Geometry check sheet. Reference: the model listing, model coordinates, mm. Round coordinates to 2 decimals unless told otherwise and drop trailing zeros. Order: outer loops, then holes, each group sorted by start corner. A loop starts at its lowest first (then second) coordinate and runs counter-clockwise, first axis right, second up. Notation, with made-up numbers: (6.25, 85) - (37.25, 85) arc R23 cw to (37.25, 113) - close; hole circle Ø1 at (-4, 59.25). An arc over 180 degrees is marked (long way). One line per question, with ' | ' between items. Start each with the question number.
Q1. Sectioned sample at C-C, the plane z = -30. Enter the section's corners in (x, y), then the cut area to 3 significant figures.
Q2. Sectioned sample at A-A, the plane z = 0. Enter the section's corners in (x, y).
Q3. Sectioned sample at B-B, the plane x = 0. Enter the section's corners in (y, z).
Q4. Material ranges on line 1 along X through (y, z) = (1.8, 0); line 2 along X through (y, z) = (7.55, 0); line 3 along Z through (x, y) = (3.5, 2.5), recorded low to high.
Q5. Sectioned sample at D-D, the plane y = 8.25. Enter the section's corners in (x, z).
Q6. Gauge pin test, flat ends, axial feed: P1, Ø1.5, axis at x = -22.5, y = 1.5, coming from the -Z side; P2, Ø4, axis at x = -14.5, y = 8, coming from the -Z side; P3, Ø1, axis at x = 32.5, y = 3, coming from the -Z side. Record the tip position at first contact, or that the pin passes through.
```python
from build123d import *

# Parameters (mm, degrees)
SKETCH_1_R          = 42.5
EXTRUDE_1_DEPTH     = 10
SKETCH_2_R          = 7
CUT_EXTRUDE_1_DEPTH = 6
SKETCH_3_R          = 2.5
CUT_EXTRUDE_2_DEPTH = 6


with BuildPart() as part:
    # Эскиз1 → Вытянуть1 (new body)
    with BuildSketch(Plane(origin=(0, 0, 0), x_dir=(1, 0, 0), z_dir=(0, 1, 0))):
        with Locations(Location((0, 0, 0), (0, 0, 270))):
            Circle(SKETCH_1_R)
    extrude(amount=EXTRUDE_1_DEPTH)

    # Эскиз2 → Вырез-Вытянуть1 (cut)
    with BuildSketch(Plane.XZ):
        with Locations(Location((-29.48960133, 0, 0), (0, 0, 270))):
            Circle(SKETCH_2_R)
        with Locations(Location((0, 29.48960133, 0), (0, 0, 270))):
            Circle(SKETCH_2_R)
        with Locations(Location((29.48960133, 0, 0), (0, 0, 270))):
            Circle(SKETCH_2_R)
        with Locations(Location((0, -29.48960133, 0), (0, 0, 270))):
            Circle(SKETCH_2_R)
    extrude(amount=-CUT_EXTRUDE_1_DEPTH, mode=Mode.SUBTRACT)

    # Эскиз3 → Вырез-Вытянуть2 (cut)
    with BuildSketch(Plane.XZ.offset(-6)):
        with Locations(Location((-29.48960133, 0, 0), (0, 0, 270))):
            Circle(SKETCH_3_R)
        with Locations(Location((0, 29.48960133, 0), (0, 0, 270))):
            Circle(SKETCH_3_R)
        with Locations(Location((29.48960133, 0, 0), (0, 0, 270))):
            Circle(SKETCH_3_R)
        with Locations(Location((0, -29.48960133, 0), (0, 0, 270))):
            Circle(SKETCH_3_R)
    extrude(amount=-CUT_EXTRUDE_2_DEPTH, mode=Mode.SUBTRACT)


solid = part.part
```
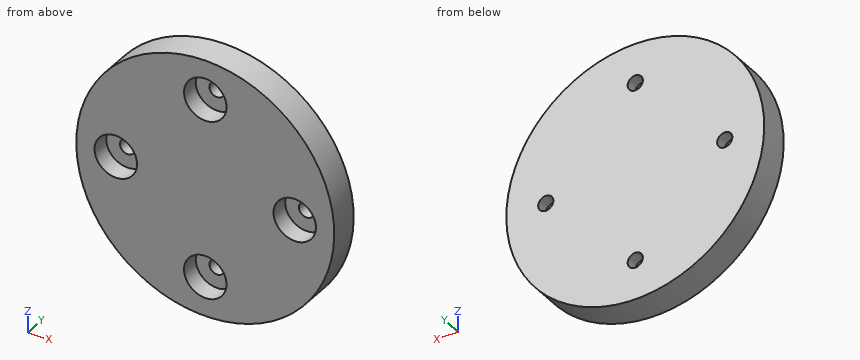
Determined:
1) outline: (-30.1, 0) - (-6.98, 0) - (-6.98, 6) - (-2.45, 6) - (-2.45, 10) - (-30.1, 10) - close; (2.45, 6) - (6.98, 6) - (6.98, 0) - (30.1, 0) - (30.1, 10) - (2.45, 10) - close | area: 499 mm2
2) outline: (-42.5, 0) - (-36.49, 0) - (-36.49, 6) - (-31.99, 6) - (-31.99, 10) - (-42.5, 10) - close; (-26.99, 6) - (-22.49, 6) - (-22.49, 0) - (22.49, 0) - (22.49, 6) - (26.99, 6) - (26.99, 10) - (-26.99, 10) - close; (31.99, 6) - (36.49, 6) - (36.49, 0) - (42.5, 0) - (42.5, 10) - (31.99, 10) - close
3) outline: (0, -42.5) - (10, -42.5) - (10, -31.99) - (6, -31.99) - (6, -36.49) - (0, -36.49) - close; (0, -22.49) - (6, -22.49) - (6, -26.99) - (10, -26.99) - (10, 26.99) - (6, 26.99) - (6, 22.49) - (0, 22.49) - close; (0, 36.49) - (6, 36.49) - (6, 31.99) - (10, 31.99) - (10, 42.5) - (0, 42.5) - close
4) line 1: x = -42.5 to -36.49, -22.49 to 22.49, 36.49 to 42.5 | line 2: x = -42.5 to -31.99, -26.99 to 26.99, 31.99 to 42.5 | line 3: z = -42.36 to -35.55, -23.43 to 23.43, 35.55 to 42.36
5) outline: circle Ø85 at (0, 0); hole circle Ø5 at (-29.49, 0); hole circle Ø5 at (0, -29.49); hole circle Ø5 at (0, 29.49); hole circle Ø5 at (29.49, 0)
6) P1: stops at z = -36.51 | P2: stops at z = -40.62 | P3: stops at z = -27.97
